Could you check a few things on this model? Use its own coordinates, in mm. Face numbers are marked on the shaded views. A direction names the side the tool comes from. Coordinates: 2 decimals unless noted, no trailing zeros. Loops run counter-clockwise (first coordinate to the right, second up) from the corner with the lowest first, then second, coordinate; pieces in that order, holes last. Notation, with made-up numbers: (33, 50.25) -> (89, 50.25) arc R16 cw to (89, 59.25) -> close; hole circle Ø10 at (15, 83.5). An arc over 180 degrees is marked (long way). One line per question, with ' | ' between items. Start each with the question number.
(1) Suppose I cut it at A-A (y = 0). Please give me the cut outline in (x, z), plus the area to 3 significant figures.
(2) If I drill on line 1 along Y through (x, z) = (0, 4); line 2 along X through (y, z) = (4.5, 4); line 3 along Y through (x, z) = (-1.5, 2), over which ranges is the centre line in solid material (lowest first)?
(3) If we mould it in two halves opening along X, with no side actions, what happens to the marked faces 1, 2, 3 and 4? For each: pulls with the +X half, pulls with the -X half, needs draft (parallel to the pull), parting line crosses it, or undercut.
(4) I'm going to push flat-ended pins straight in: pin 1 Ø1.8 at (y, z) = (-1, 8.5) entering from -X; pin 2 Ø1.5 at (x, z) = (4, 3) entering from +Y; pin 3 Ø5 at (y, z) = (-4.5, 8) entering from +X. Where does each tip first touch, or does it pass through?
(5) Suppose I cut it at B-B (x = -2.75). Please give me the cut outline in (y, z).
(6) Which directions (+Z, -Z, +X, -X, +Y, -Y) give clear straight access to the entire face, cutting with the end or side of a thin tool? Please do the marked faces 5 and 6.
(7) Suppose I cut it at D-D (x = 0). Please give me the cut outline in (y, z).
(8) Suppose I cut it at C-C (z = 10.25). Please give me the cut outline in (x, y), plus the area to 3 significant figures.
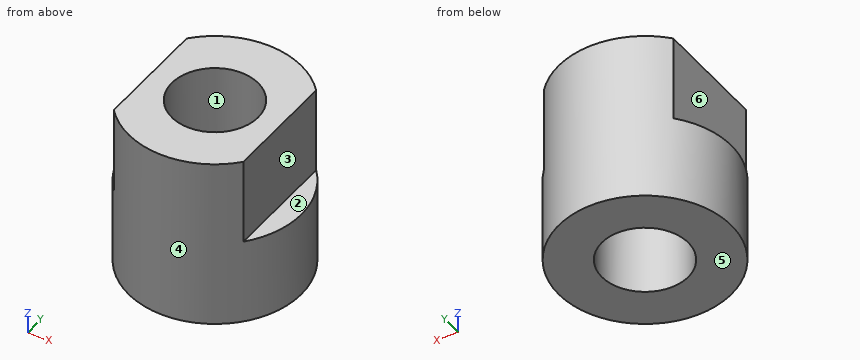
Autodesk Fusion 360 part; units mm, degrees
sketch "Esquisse1" plane through (0, 0, 0) normal (0, 0, 1) x (1, 0, 0)
  circle A0 centre (0, 0) radius 3
  circle A1 centre (0, 0) radius 6
  line L0 (-4.5, 8.8472) -> (4.5, 8.8472) construction
  line L1 (4.5, 8.8472) -> (4.5, -9.3481) construction
  line L2 (4.5, -9.3481) -> (-4.5, -9.3481) construction
  line L3 (-4.5, -9.3481) -> (-4.5, 8.8472) construction
  line L4 (4.5, 3.9686) -> (4.5, -3.9686)
  line L5 (-4.5, 3.9686) -> (-4.5, -3.9686)
  dimension "d1" = 6
  dimension "d2" = 12
  dimension "d3" = 9
  dimension "d4" = 4.5
extrude "Extrusion3" add sketch "Esquisse1" along normal blind 12
sketch "Esquisse2" plane through (0, 0, 12) normal (0, 0, 1) x (-1, 0, 0)
  circle A0 centre (0, 0) radius 3
  circle A1 centre (0, 0) radius 6
  line L0 (4.5, -8.2141) -> (-4.5, -8.2141) construction
  line L1 (-4.5, -8.2141) -> (-4.5, 8.5) construction
  line L2 (-4.5, 8.5) -> (4.5, 8.5) construction
  line L3 (4.5, 8.5) -> (4.5, -8.2141) construction
  line L4 (4.5, 3.9686) -> (4.5, -3.9686)
  line L5 (-4.5, -3.9686) -> (-4.5, 3.9686)
  dimension "d12" = 9
  dimension "d13" = 4.5
extrude "Extrusion4" cut sketch "Esquisse2" against normal blind 6 contours A1 L4 | A1 L5
Checks:
1) outline: (-6, 0) -> (-3, 0) -> (-3, 12) -> (-4.5, 12) -> (-4.5, 6) -> (-6, 6) -> close; (3, 0) -> (6, 0) -> (6, 6) -> (4.5, 6) -> (4.5, 12) -> (3, 12) -> close | area: 54.0 mm^2
2) line 1: y = -6 to -3, 3 to 6 | line 2: x = -3.97 to 3.97 | line 3: y = -5.81 to -2.6, 2.6 to 5.81
3) face 1: undercut | face 2: needs draft | face 3: pulls with the +X half | face 4: parting line crosses it
4) pin 1: stops at x = -4.5 | pin 2: stops at y = 5.04 | pin 3: stops at x = 5.2
5) outline: (-5.33, 0) -> (-1.2, 0) -> (-1.2, 12) -> (-5.33, 12) -> close; (1.2, 0) -> (5.33, 0) -> (5.33, 12) -> (1.2, 12) -> close
6) face 5: -Z, +X, -X, +Y, -Y | face 6: +Z, -X, +Y, -Y
7) outline: (-6, 0) -> (-3, 0) -> (-3, 12) -> (-6, 12) -> close; (3, 0) -> (6, 0) -> (6, 12) -> (3, 12) -> close
8) outline: (-4.5, -3.97) arc R6 ccw to (4.5, -3.97) -> (4.5, 3.97) arc R6 ccw to (-4.5, 3.97) -> close; hole circle Ø6 at (0, 0) | area: 68.5 mm^2
